Design review of the part built by this model. Coordinates are the model's own, in mm. Give positions to 0.01 mm unless a question says otherwise; leave off trailing zeros. Order: outer loops, then holes, each group sorted by start corner. A loop starts at its lowest first (then second) coordinate and runs counter-clockwise, first axis right, second up. Notation, with made-up numbers: M -33,81.25 L -23,81.25 A9 ccw -23,90.25 Z; hole C 11.5,70 d11. An arc over 180 degrees is marked long. Answer as a JSON object with one key per item and string values.
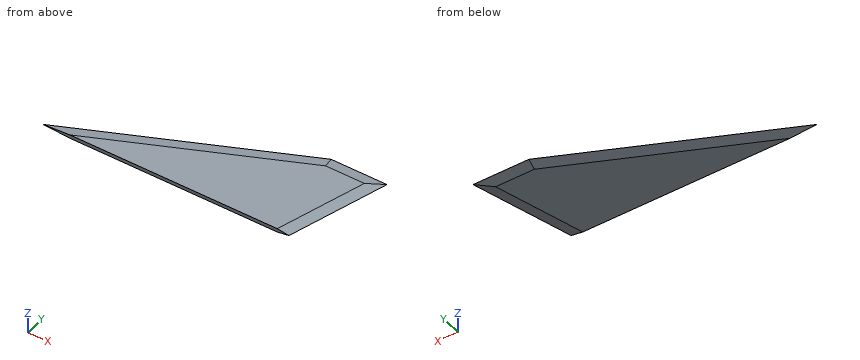
from build123d import *
from OCP.BRepFilletAPI import BRepFilletAPI_MakeChamfer

# Parameters (mm, degrees)
BOSS_EXTRUDE1_DEPTH = 1.59
CHAMFER1_SIZE       = 1.59
CHAMFER1_SIZE2      = 10
CHAMFER2_SIZE       = 10
CHAMFER2_SIZE_2     = 1.59
SKETCH2_R           = 41
CUT_EXTRUDE1_DEPTH  = 220


with BuildPart() as part:
    # Sketch1 → Boss-Extrude1 (new, symmetric)
    with BuildSketch(Plane.XY):
        Polygon((0, 0), (220, 0), (245, 88.9), (195, 88.9), align=None)
    extrude(amount=BOSS_EXTRUDE1_DEPTH, both=True)

    # Chamfer1: one chamfer whose edges measure the first distance from different faces: ONE call of the kernel's chamfer builder (chamfer() names one face for all edges)
    chamfer1_edges_1 = [part.edges().sort_by_distance(p)[0] for p in [
        (232.5, 44.45, 1.59),
    ]]
    chamfer1_side_1 = [part.faces().sort_by_distance(p)[0] for p in [
        (232.5, 44.45, 0),
    ]]
    chamfer1_edges_2 = [part.edges().sort_by_distance(p)[0] for p in [
        (220, 88.9, 1.59),
    ]]
    chamfer1_side_2 = [part.faces().sort_by_distance(p)[0] for p in [
        (220, 88.9, 0),
    ]]
    chamfer1_edges_3 = [part.edges().sort_by_distance(p)[0] for p in [
        (97.5, 44.45, 1.59),
    ]]
    chamfer1_side_3 = [part.faces().sort_by_distance(p)[0] for p in [
        (97.5, 44.45, 0),
    ]]
    chamfer1 = BRepFilletAPI_MakeChamfer(part.part.solid().wrapped)
    for e in chamfer1_edges_1:
        chamfer1.Add(CHAMFER1_SIZE, CHAMFER1_SIZE2, e.wrapped, chamfer1_side_1[0].wrapped)  # the first distance lies on this face
    for e in chamfer1_edges_2:
        chamfer1.Add(CHAMFER1_SIZE, CHAMFER1_SIZE2, e.wrapped, chamfer1_side_2[0].wrapped)  # the first distance lies on this face
    for e in chamfer1_edges_3:
        chamfer1.Add(CHAMFER1_SIZE, CHAMFER1_SIZE2, e.wrapped, chamfer1_side_3[0].wrapped)  # the first distance lies on this face
    add(Compound.cast(chamfer1.Shape()), mode=Mode.REPLACE)

    # Chamfer2
    # the kernel refuses this chamfer: 10, 1.59 mm, written as the material it takes off along each edge
    with BuildSketch(Plane(origin=(218.64660826, 99.680428074, -1.59), x_dir=(0.41481463774773214, -0.9098858758246093, -0.006042291378384615), z_dir=(-0.9099024859208529, -0.41482221024801963, 0))) as chamfer2_piece_1:
        Polygon((CHAMFER2_SIZE * 0.999981745191, CHAMFER2_SIZE * 0.00604229137838), (-CHAMFER2_SIZE_2 * 0.00604229137839, CHAMFER2_SIZE_2 * 0.999981745191), (0, 0), align=None)
    extrude(amount=266.284816527, mode=Mode.SUBTRACT)
    with BuildSketch(Plane(origin=(270.98806864, 88.9, -1.59), x_dir=(0, -0.9999817451908304, -0.006042291378384616), z_dir=(-1, 0, 0))) as chamfer2_piece_2:
        Polygon((CHAMFER2_SIZE * 0.999981745191, CHAMFER2_SIZE * 0.00604229137838), (-CHAMFER2_SIZE_2 * 0.00604229137838, CHAMFER2_SIZE_2 * 0.999981745191), (0, 0), align=None)
    extrude(amount=101.976137281, mode=Mode.SUBTRACT)
    with BuildSketch(Plane(origin=(212.96466032, -25.017667902, -1.59), x_dir=(0.22378185481817084, -0.06293078032007055, 0.9726054690070615), z_dir=(0.2707142180235852, 0.9626597592918689, 0))) as chamfer2_piece_3:
        Polygon((CHAMFER2_SIZE_2 * 0.972605469007, -CHAMFER2_SIZE_2 * 0.232462043477), (-CHAMFER2_SIZE * 0.232462043477, -CHAMFER2_SIZE * 0.972605469007), (0, 0), align=None)
    extrude(amount=144.324445333, mode=Mode.SUBTRACT)

    # Sketch2 → Cut-Extrude1 (cut)
    with BuildSketch(Plane(origin=(0, 0, 0), x_dir=(0, 0, -1), z_dir=(1, 0, 0))):
        with Locations((0, -40.969157912)):
            Circle(SKETCH2_R)
    extrude(amount=CUT_EXTRUDE1_DEPTH, mode=Mode.SUBTRACT)


solid = part.part
(1) To check wall thickness, follow L1, parallel to Z at x = 235, y = 85.5. State the ranges of the line that lie inside material, in increasing order. Write a range as from..to.
Checked values:
{"L1": "z = -0.54..0.54"}
(2) We need section D-D (x = 110.5). Write out the cut boundary in (y, z).
Checked values:
{"outline": "M 0,-1.59 L 39.39,-1.59 L 50.38,0 L 39.39,1.59 L 0,1.59 A41 cw Z"}
(3) We need section A-A (y = 42). Write out the cut boundary in (x, z).
Checked values:
{"outline": "M 92.13,0 L 116.23,-1.59 L 221.42,-1.59 L 231.81,0 L 221.42,1.59 L 116.23,1.59 Z"}
(4) We need section C-C (z = -0.8). Write out the cut boundary in (x, y).
Checked values:
{"outline": "M 12.18,0.02 L 214.78,0.02 L 238.36,83.87 L 196.09,83.87 Z"}
(5) We need section B-B (x = 228.5). Write out the cut boundary in (y, z), plus the area to 3 significant figures.
Checked values:
{"outline": "M 30.23,0 L 67.17,-1.59 L 78.9,-1.59 L 88.9,0 L 78.9,1.59 L 67.17,1.59 Z", "area": "112 mm^2"}
